Study the drawing (mm; zero at the part's minimum x, y, z) and answer. Coordinates: 2 decimals unless noted, no trailing zeros. Loops run counter-clockwise (first coordinate to the right, second up) from the corner with the lowest first, then second, coordinate; pieces in that order, holes last. Notation, with made-up numbers: (-11, 51.25) -> (29, 51.25) arc R8 ccw to (29, 58.25) -> close; hole circle Ø5 at (88.5, -16.5). An arc over 180 degrees is marked (long way). Answer as a JSON object with one key per item and string values. Group by question number.
Q1. The part is cut by section A-A on z = 1.9. Write down the section's boundary in (x, y) (3 decimals).
Q2. The part is cut by section B-B on x = 130. Write down the section's boundary in (y, z) (3 decimals), and give its area (3 significant figures).
Q3. The part is cut by section C-C on y = 20. Write down the section's boundary in (x, z) (3 decimals).
Q4. Each of these flat-tipped pins is pushed along its axis until it touches: P1, Ø1, axis at x = 2, z = 1, coming from the +Y side; P2, Ø1, axis at y = 78, z = 1, coming from the -X side (3 decimals); P3, Ø1, axis at x = 137, z = 1.5, coming from the +Y side (3 decimals). Where does it stop, or does it pass through?
Q5. Straight lines are drawn through the part: line 1 along Y through (x, z) = (118, 2.7) (3 decimals); line 2 along X through (y, z) = (75, 0.3) (3 decimals). For each, find the intervals that lie inside material, in ascending order. Write a range as [from, to].
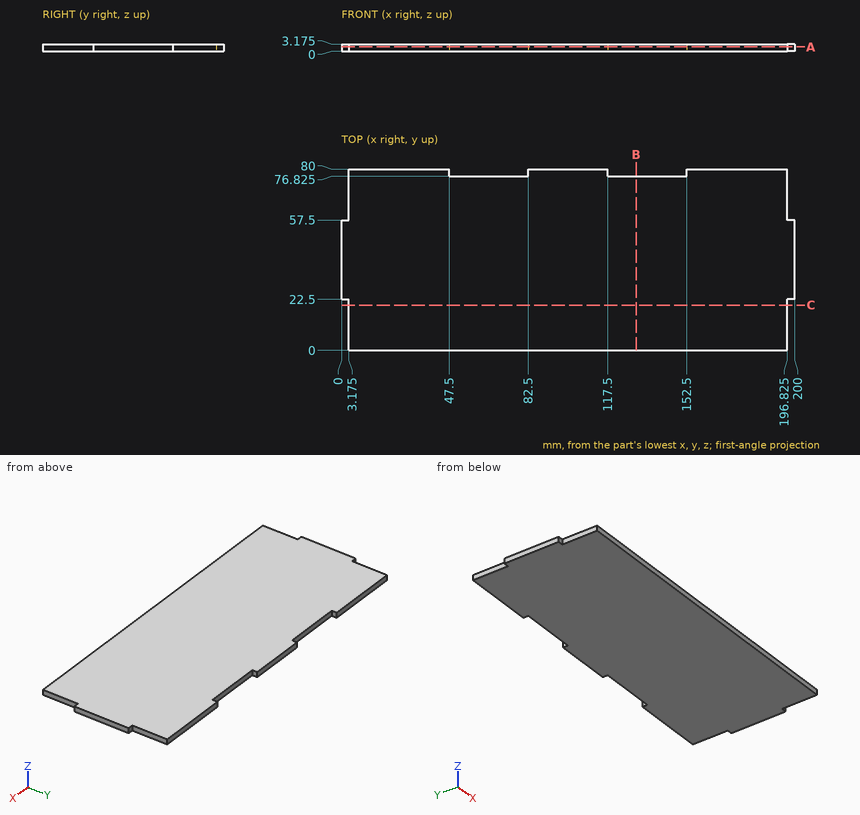
Final values:
{
 "1": {"outline": "(0, 22.5) -> (3.175, 22.5) -> (3.175, 0) -> (196.825, 0) -> (196.825, 22.5) -> (200, 22.5) -> (200, 57.5) -> (196.825, 57.5) -> (196.825, 80) -> (152.5, 80) -> (152.5, 76.825) -> (117.5, 76.825) -> (117.5, 80) -> (82.5, 80) -> (82.5, 76.825) -> (47.5, 76.825) -> (47.5, 80) -> (3.175, 80) -> (3.175, 57.5) -> (0, 57.5) -> close"},
 "2": {"outline": "(0, 0) -> (76.825, 0) -> (76.825, 3.175) -> (0, 3.175) -> close", "area": "244 mm2"},
 "3": {"outline": "(3.175, 0) -> (196.825, 0) -> (196.825, 3.175) -> (3.175, 3.175) -> close"},
 "4": {"P1": "stops at y = 57.5", "P2": "stops at x = 3.175", "P3": "stops at y = 76.825"},
 "5": {"line 1": "y = [0, 76.825]", "line 2": "x = [3.175, 196.825]"}
}
